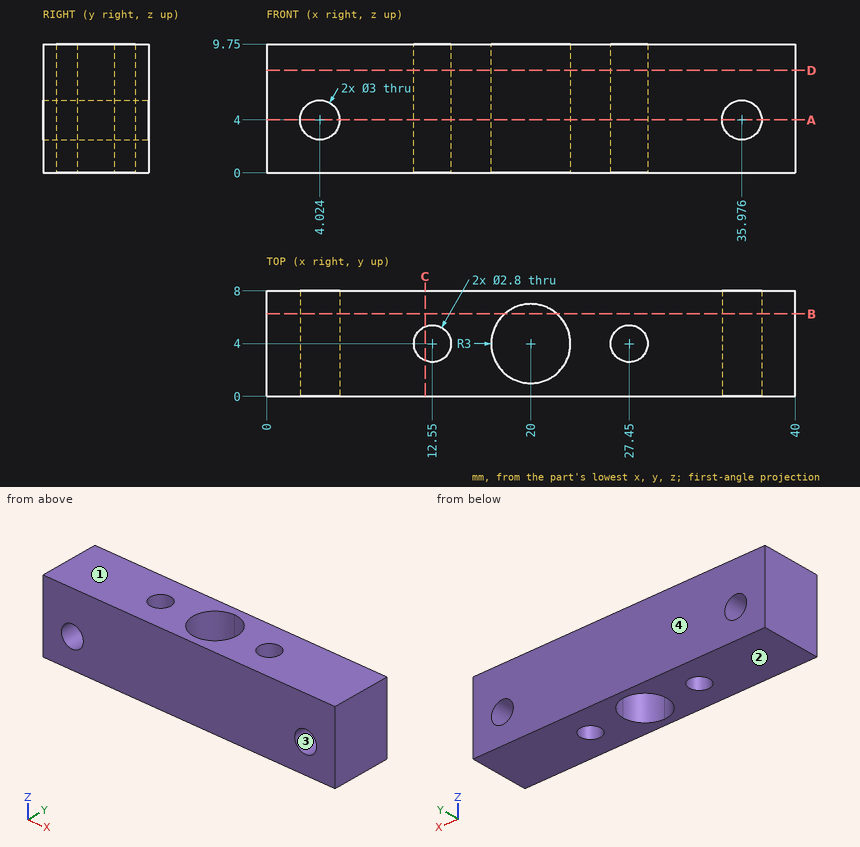
Could you check a few things on this drawing? It's one solid part, dimensions in mm from its lowest x, y, z. Round coordinates to 2 decimals unless told otherwise and drop trailing zeros. Order: outer loops, then holes, each group sorted by start corner. A loop starts at its lowest first (then second) coordinate and runs counter-clockwise, first axis right, second up. Notation, with made-up numbers: M 52,44 L 77,44 A8 ccw 77,50 Z; hole C 20.5,33.5 d8. An arc over 180 degrees is marked long. One line per question, with ' | ' between items.
1) I need wall thicknesses on line 1 (X direction, y = 4.5, z = 5); line 2 (Z direction, x = 36.5, y = 2.5); line 3 (X direction, y = 2.75, z = 3.75) (1 decimal). Which ranges of each line are inside material? Lowest first, please.
Checked values:
line 1: x = 0 to 2.91, 5.14 to 11.24, 13.86 to 17.04, 22.96 to 26.14, 28.76 to 34.86, 37.09 to 40 | line 2: z = 0 to 2.59, 5.41 to 9.75 | line 3: x = 0 to 2.5, 5.5 to 11.9, 13.2 to 17.3, 22.7 to 26.8, 28.1 to 34.5, 37.5 to 40
2) Imagine slicing it at B-B, the plane y = 6.25. Write out the boundary of the cut face in (x, z).
Checked values:
outline: M 0,0 L 18.02,0 L 18.02,9.75 L 0,9.75 Z; M 21.98,0 L 40,0 L 40,9.75 L 21.98,9.75 Z; hole C 4.02,4 d3; hole C 35.98,4 d3
3) Imagine slicing it at C-C, the plane x = 12. Write out the boundary of the cut face in (y, z).
Checked values:
outline: M 0,0 L 2.71,0 L 2.71,9.75 L 0,9.75 Z; M 5.29,0 L 8,0 L 8,9.75 L 5.29,9.75 Z
4) Imagine slicing it at A-A, the plane z = 4. Write out the boundary of the cut face in (x, y), plus the area to 3 significant figures.
Checked values:
outline: M 0,0 L 2.52,0 L 2.52,8 L 0,8 Z; M 5.52,0 L 34.48,0 L 34.48,8 L 5.52,8 Z; M 37.48,0 L 40,0 L 40,8 L 37.48,8 Z; hole C 12.55,4 d2.8; hole C 20,4 d6; hole C 27.45,4 d2.8 | area: 231 mm²
5) We'd pull the mould along Z, two halves only. Please class the marked faces 1, 2, 3 and 4: released by +Z, released by -Z, zero draft, split by the parting line, or undercut.
Checked values:
face 1: released by +Z | face 2: released by -Z | face 3: undercut | face 4: zero draft
6) Imagine slicing it at D-D, the plane z = 7.75. Write out the boundary of the cut face in (x, y), plus the area to 3 significant figures.
Checked values:
outline: M 0,0 L 40,0 L 40,8 L 0,8 Z; hole C 12.55,4 d2.8; hole C 20,4 d6; hole C 27.45,4 d2.8 | area: 279 mm²
